from build123d import *

# Parameters (mm, degrees)
SKETCH1_W                      = 120
SKETCH1_H                      = 42.5
BOSS_EXTRUDE1_DEPTH            = 7
SKETCH2_R                      = 9.5
CUT_EXTRUDE1_DEPTH             = 10.6
SKETCH3_R                      = 6.5
CUT_EXTRUDE2_DEPTH             = 65.528462712
SKETCH5_R                      = 6
CUT_EXTRUDE4_DEPTH             = 66.173326599
M5X0_8_TAPPED_HOLE1_AT_2_COUNT = 2
M5X0_8_TAPPED_HOLE1_AT_2_PITCH = 28
SKETCH19_R                     = 1.25
CUT_EXTRUDE7_DEPTH             = 10
M5X0_8_TAPPED_HOLE2_REACH      = 75.86
M5X0_8_TAPPED_HOLE2_BORE_R     = 2.1
SKETCH14_W                     = 14
SKETCH14_H                     = 42.5
BOSS_EXTRUDE2_DEPTH            = 11
SKETCH15_W                     = 11
SKETCH15_H                     = 30
CUT_EXTRUDE5_DEPTH             = 7
SKETCH16_W                     = 10
SKETCH16_H                     = 14
CUT_EXTRUDE6_DEPTH             = 75.441671835
FILLET1_R                      = 3
M3X0_5_TAPPED_HOLE1_D          = 2.5
CHAMFER1_SIZE                  = 0.5


with BuildPart() as part:
    # Sketch1 → Boss-Extrude1 (new, symmetric)
    with BuildSketch(Plane.XY):
        Rectangle(SKETCH1_W, SKETCH1_H)
    extrude(amount=BOSS_EXTRUDE1_DEPTH, both=True)

    # Sketch2 → Cut-Extrude1 (cut)
    with BuildSketch(Plane.XY.offset(7)):
        Circle(SKETCH2_R)
    extrude(amount=-CUT_EXTRUDE1_DEPTH, mode=Mode.SUBTRACT)

    # Sketch3 → Cut-Extrude2 (cut, through all)
    with BuildSketch(Plane.XY.offset(-3.6)):
        Circle(SKETCH3_R)
    extrude(amount=-CUT_EXTRUDE2_DEPTH, mode=Mode.SUBTRACT)

    # Sketch5 → Cut-Extrude4 (cut, through all)
    with BuildSketch(Plane.XY.offset(7)):
        with Locations((-50, 3.4)):
            Circle(SKETCH5_R)
        with Locations((50, 3.4)):
            Circle(SKETCH5_R)
    extrude(amount=-CUT_EXTRUDE4_DEPTH, mode=Mode.SUBTRACT)

    # Sketch8 → M5x0.8 Tapped Hole1 (revolve, cut)
    with BuildSketch(Plane(origin=(-22, -21.25, 0), x_dir=(0, 0, -1), z_dir=(1, 0, 0))):
        Polygon((0, 0), (0, 12.0618073), (2.1, 10.8), (2.1, 0), align=None)
    m5x0_8_tapped_hole1 = revolve(axis=Axis((-22, -27.6, 0), (0, 1, 0)), mode=Mode.SUBTRACT)

    # M5x0.8 Tapped Hole1 at 2: M5x0.8 Tapped Hole1 ×2
    with Locations(*[(-i * M5X0_8_TAPPED_HOLE1_AT_2_PITCH, 0, 0) for i in range(1, M5X0_8_TAPPED_HOLE1_AT_2_COUNT)]):
        add(m5x0_8_tapped_hole1, mode=Mode.SUBTRACT)

    # Sketch19 → Cut-Extrude7 (cut)
    with BuildSketch(Plane.XZ.offset(21.25)):
        with Locations(Location((-36, 0, 0), (0, 0, 270))):
            Circle(SKETCH19_R)
    cut_extrude7 = extrude(amount=-CUT_EXTRUDE7_DEPTH, mode=Mode.SUBTRACT)

    # Mirror1: M5x0.8 Tapped Hole1, Cut-Extrude7 across plane
    add(m5x0_8_tapped_hole1.mirror(Plane(origin=(0, 0, 0), x_dir=(0, 0, 1), z_dir=(1, 0, 0))), mode=Mode.SUBTRACT)
    add(cut_extrude7.mirror(Plane(origin=(0, 0, 0), x_dir=(0, 0, 1), z_dir=(1, 0, 0))), mode=Mode.SUBTRACT)

    # Mirror1 copy 1 sketch → Mirror1 copy 1 (revolve, cut)
    with BuildSketch(Plane(origin=(50, -21.25, 0), x_dir=(0, 0, -1), z_dir=(-1, 0, 0))):
        Polygon((0, 0), (0, -12.0618073), (2.1, -10.8), (2.1, 0), align=None)
    revolve(axis=Axis((50, -27.6, 0), (0, -1, 0)), mode=Mode.SUBTRACT)

    # M5x0.8 Tapped Hole2 bore → M5x0.8 Tapped Hole2 (cut, up to next)
    with BuildSketch(Plane(origin=(0, 21.25, 0), x_dir=(1, 0, 0), z_dir=(0, 1, 0)), mode=Mode.PRIVATE) as m5x0_8_tapped_hole2_sk1:
        with Locations((-50, 0)):
            Circle(M5X0_8_TAPPED_HOLE2_BORE_R)
    m5x0_8_tapped_hole2_tool1 = extrude(m5x0_8_tapped_hole2_sk1.sketch, amount=-M5X0_8_TAPPED_HOLE2_REACH, mode=Mode.PRIVATE) & part.part
    # M5x0.8 Tapped Hole2 bore → M5x0.8 Tapped Hole2 (cut, up to next)
    with BuildSketch(Plane(origin=(0, 21.25, 0), x_dir=(1, 0, 0), z_dir=(0, 1, 0)), mode=Mode.PRIVATE) as m5x0_8_tapped_hole2_sk2:
        with Locations((50, 0)):
            Circle(M5X0_8_TAPPED_HOLE2_BORE_R)
    m5x0_8_tapped_hole2_tool2 = extrude(m5x0_8_tapped_hole2_sk2.sketch, amount=-M5X0_8_TAPPED_HOLE2_REACH, mode=Mode.PRIVATE) & part.part
    add(m5x0_8_tapped_hole2_tool1.solids().sort_by_distance((-50, 21.25, 0))[0], mode=Mode.SUBTRACT)
    add(m5x0_8_tapped_hole2_tool2.solids().sort_by_distance((50, 21.25, 0))[0], mode=Mode.SUBTRACT)

    # Sketch14 → Boss-Extrude2 (add)
    with BuildSketch(Plane(origin=(60, 0, 0), x_dir=(0, 0, -1), z_dir=(1, 0, 0))):
        Rectangle(SKETCH14_W, SKETCH14_H)
    extrude(amount=BOSS_EXTRUDE2_DEPTH)

    # Sketch15 → Cut-Extrude5 (cut)
    with BuildSketch(Plane.XY.offset(7)):
        with Locations((65.5, 2)):
            Rectangle(SKETCH15_W, SKETCH15_H)
    extrude(amount=-CUT_EXTRUDE5_DEPTH, mode=Mode.SUBTRACT)

    # Sketch16 → Cut-Extrude6 (cut, through all)
    with BuildSketch(Plane.XY):
        with Locations((66, 2)):
            Rectangle(SKETCH16_W, SKETCH16_H)
    extrude(amount=-CUT_EXTRUDE6_DEPTH, mode=Mode.SUBTRACT)

    # Fillet1
    fillet1_edges = [part.edges().sort_by_distance(p)[0] for p in [
        (61, -5, -3.5),
        (61, 9, -3.5),
        (60, -13, 3.5),
        (60, 17, 3.5),
    ]]
    fillet(fillet1_edges, radius=FILLET1_R)

    # M3x0.5 Tapped Hole1 (through all)
    with Locations(Plane.XY):
        with Locations((65.5, 12), (65.5, -8)):
            Hole(M3X0_5_TAPPED_HOLE1_D / 2)

    # Chamfer1
    chamfer1_edges = [part.edges().sort_by_distance(p)[0] for p in [
        (-60, 0, 7),
        (71, 9, -3.5),
        (71, -5, -3.5),
        (67.5, 9, -7),
        (67.5, 9, 0),
        (67.5, -5, 0),
        (67.5, -5, -7),
        (61, 2, 0),
        (61, 2, -7),
        (67, -13, 7),
        (60, 2, 7),
        (61.878679656, -4.121320344, 0),
        (61.878679656, -4.121320344, -7),
        (60.878679656, -12.121320344, 7),
        (60.878679656, 16.121320344, 7),
        (61.878679656, 8.121320344, 0),
        (61.878679656, 8.121320344, -7),
        (5.5, -21.25, 7),
        (-9.5, 0, 7),
        (-6.5, 0, -7),
        (-6.5, 0, -3.6),
        (-56, 3.4, -7),
        (-56, 3.4, 7),
        (44, 3.4, -7),
        (44, 3.4, 7),
        (5.5, -21.25, -7),
        (-60, 0, -7),
        (5.5, 21.25, -7),
        (5.5, 21.25, 7),
        (71, 19.125, 7),
        (71, -21.25, 0),
        (71, -13.125, -7),
        (71, 21.25, 0),
        (-60, -21.25, 0),
        (-60, 21.25, 0),
        (71, -17.125, 7),
        (71, -9, 0),
        (71, 17, 3.5),
        (71, -13, 3.5),
        (67, 17, 7),
        (71, 13, 0),
        (71, 15.125, -7),
    ]]
    chamfer(chamfer1_edges, length=CHAMFER1_SIZE)


solid = part.part
Work out the finished part from the listing and answer in its coordinate system (mm). A direction names the side the tool comes from. Round coordinates to 2 decimals unless told otherwise and drop trailing zeros. Order: outer loops, then holes, each group sorted by start corner. A loop starts at its lowest first (then second) coordinate and runs counter-clockwise, first axis right, second up. Notation, with made-up numbers: M 46,18.25 L 86,18.25 A30 ccw 86,44.25 Z; hole C 21.25,-35 d1. An arc over 180 degrees is marked long. Put each result on its own line as item: value. Start each with the question number.
Q1. Section C-C, the plane x = 0 is taken. Write down the section's boundary in (y, z).
Q2. Section A-A, the plane x = 65.5 is taken. Give the number of separate pieces and of enclosed holes in the cut face, and give its area (3 significant figures).
Q3. Flat-ended cylindrical pins translate along their axes: pin 1 (2.5 mm diameter, centred on x = 50, z = 0, fed in from -Y); pin 2 (11.5 mm diameter, centred on x = 66.5, y = 8, fed in from +Z); pin 3 (6.5 mm diameter, centred on y = 2.5, z = -2.5, fed in from +X). Find the tip coordinate at first contact, or state that the pin passes through.
Q4. Section D-D, the plane x = 36 is taken. Write down the section's boundary in (y, z), and give its area (4 significant figures).
Q5. For a pull along Y with two mould halves and no side action, classify faces 1 (the flat face through (36, -11.25, 0)), 2 (the conical face through (60.807, 16.241, 6.635)), 3 (the flat face through (-60, 0, 0)) as pulls with the +Y half, pulls with the -Y half, needs draft (parallel to the pull), parting line crosses it, or undercut.
Q6. A tool of negligible diameter and unlimited length cuts with its end or side. For faces 4 (the cylindrical face through (4.38, -8.43, 1.52)), 5 (the cylindrical face through (-23.77, -15.93, -1.13)), 6 (the cylindrical face through (51.94, 15.22, 0.8)), 7 (the cylindrical face through (60.9, 16.14, 3.2)), 8 (the flat face through (5, -21.25, 0)), from which of +Z, -Z, +X, -X, +Y, -Y can it reach the whole face along a straight path? Write none if from no direction.
Q7. Section B-B, the plane y = -17.5 is taken. Write down the section's boundary in (x, z).
Q8. Straight lines are drawn through the part: L1, parallel to X at y = 6, z = 4.5; L2, parallel to X at y = 1, z = 4; L3, parallel to Z at x = -50, y = 14.5. For each, find the intervals that lie inside material, in ascending order. Write a range as [from, to].
Findings below:
1. outline: M -21.25,-6.5 L -20.75,-7 L -7,-7 L -6.5,-6.5 L -6.5,-4.1 L -7,-3.6 L -9.5,-3.6 L -9.5,6.5 L -10,7 L -20.75,7 L -21.25,6.5 Z; M 6.5,-6.5 L 7,-7 L 20.75,-7 L 21.25,-6.5 L 21.25,6.5 L 20.75,7 L 10,7 L 9.5,6.5 L 9.5,-3.6 L 7,-3.6 L 6.5,-4.1 Z
2. separate pieces: 4
2. enclosed holes: 0
2. area: 251 mm^2
3. pin 1: stops at y = -9.94
3. pin 2: stops at z = 0
3. pin 3: stops at x = 61
4. outline: M -21.25,-6.5 L -20.75,-7 L 20.75,-7 L 21.25,-6.5 L 21.25,6.5 L 20.75,7 L -20.75,7 L -21.25,6.5 L -21.25,1.25 L -11.25,1.25 L -11.25,-1.25 L -21.25,-1.25 Z
4. area: 569.5 mm^2
5. face 1: pulls with the -Y half
5. face 2: undercut
5. face 3: needs draft
6. face 4: +Z
6. face 5: -Y
6. face 6: +Y
6. face 7: +Z, +X
6. face 8: +Z, -Z, +X, -X, -Y
7. outline: M -60,-6.5 L -59.5,-7 L 70.5,-7 L 71,-6.5 L 71,6.5 L 70.5,7 L -59.5,7 L -60,6.5 Z; hole C -50,0 d4.2; hole C -36,0 d2.5; hole C -22,0 d4.2; hole C 22,0 d4.2; hole C 36,0 d2.5; hole C 50,0 d4.2
8. L1: x = [-60, -55.41], [-44.59, -7.37], [7.37, 44.59], [55.41, 60]
8. L2: x = [-60, -55.5], [-44.5, -9.45], [9.45, 44.5], [55.5, 60]
8. L3: z = [-7, -2.1], [2.1, 7]
